Build history of the part. All positions in model axes, mm. Face numbers are marked on the shaded views. A direction names the side the tool comes from. Round coordinates to 2 decimals unless told otherwise and drop trailing zeros. Loops run counter-clockwise (first coordinate to the right, second up) from the corner with the lowest first, then second, coordinate; pieces in that order, holes last. Notation, with made-up numbers: (-11, 24) -> (41, 24) arc R35 cw to (41, 59) -> close; hole circle Ø8 at (-27, 84.25). An arc over 180 degrees is marked (long way). Put each result on its own line as item: value. Start each with the question number.
Item 1: Cut at B-B, the plane x = 156.5. List the corners of the cut face in (y, z), plus the area to 3 significant figures.
Item 2: Cut at A-A, the plane y = 334. List the corners of the cut face in (x, z), plus the area to 3 significant figures.
Item 3: Cut at C-C, the plane z = 1.45. List the corners of the cut face in (x, y).
Item 4: Tool access for the marked faces 1 and 2: list every direction of +Z, -Z, +X, -X, +Y, -Y with a clear straight run to the whole face (end or side of a thin tool).
Item 5: Cut at D-D, the plane y = 355. List the corners of the cut face in (x, z).
Item 6: Flat gauge pins, fed straight in: pin 1 Ø8 at (x, y) = (145.5, 366) entering from +Z; pin 2 Ø1.5 at (y, z) = (352.5, 0.5) entering from -X; pin 3 Ø1.5 at (x, z) = (157, 0.5) entering from +Y. Where does each tip first touch, or does it go through?
Item 7: Drill centre lines: probe 1 along X at (y, z) = (363, 0.35); probe 2 along Z at (x, y) = (118, 332.5); probe 3 along X at (y, z) = (361.5, 1.6). Where is each one in solid material? Low to high. Write a range as [from, to].
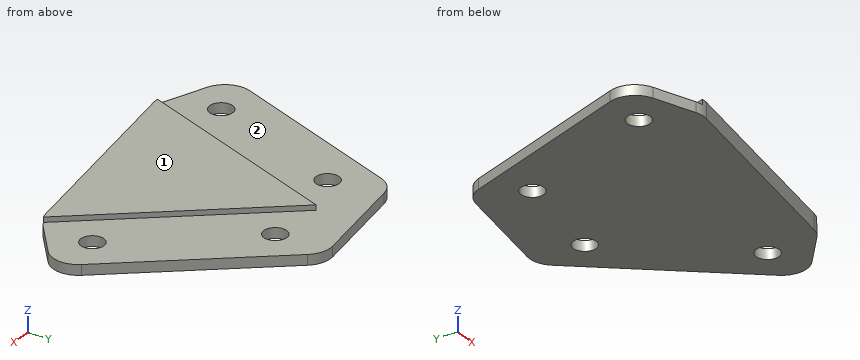
```python
from build123d import *

# Parameters (mm, degrees)
EXTRUDE_1_DEPTH     = 3
SKETCH_2_R          = 2.25
CUT_EXTRUDE_1_DEPTH = 3
FILLET_1_R          = 5
CUT_EXTRUDE_2_DEPTH = 1


with BuildPart() as part:
    # ｽｹｯﾁ1 → ﾎﾞｽ - 押し出し1 (new body)
    with BuildSketch(Plane.XY):
        Polygon((173.531323483, 340.900859956), (144.605881047, 375.372859896), (133.1152144, 365.731045751), (119.019825089, 370.861347901), (103.628918639, 328.575179965), (117.724307951, 323.444877815), (162.040656836, 331.259045811), align=None)
        Polygon((144.605881047, 375.372859896), (133.1152144, 365.731045751), (119.019825089, 370.861347901), align=None)
    extrude(amount=EXTRUDE_1_DEPTH)

    # ｽｹｯﾁ2 → ｶｯﾄ - 押し出し1 (cut)
    with BuildSketch(Plane.XY.offset(3)):
        with Locations((113.24176437, 333.057723546)):
            Circle(SKETCH_2_R)
        with Locations((123.50236867, 361.24850217)):
            Circle(SKETCH_2_R)
        with Locations((143.681454796, 364.8066195)):
            Circle(SKETCH_2_R)
        with Locations((162.965083087, 341.825286207)):
            Circle(SKETCH_2_R)
    extrude(amount=-CUT_EXTRUDE_1_DEPTH, mode=Mode.SUBTRACT)

    # ﾌｨﾚｯﾄ1
    fillet_1_edges = [part.edges().sort_by_distance(p)[0] for p in [
        (173.531323483, 340.900859956, 1.5),
        (162.040656836, 331.259045811, 1.5),
        (117.724307951, 323.444877815, 1.5),
        (103.628918639, 328.575179965, 1.5),
        (119.019825089, 370.861347901, 1.5),
        (144.605881047, 375.372859896, 1.5),
    ]]
    fillet(fillet_1_edges, radius=FILLET_1_R)

    # ｽｹｯﾁ3 → ｶｯﾄ - 押し出し2 (cut)
    with BuildSketch(Plane.XY.offset(3)):
        Polygon((121.413966092, 377.439196246), (103.628918639, 328.575179965), (117.771292582, 323.427776808), (133.132579218, 365.632564976), (162.002354614, 331.22690643), (173.531323483, 340.900859956), (140.106367779, 380.735170998), (131.711632891, 373.691152049), align=None)
    extrude(amount=-CUT_EXTRUDE_2_DEPTH, mode=Mode.SUBTRACT)


solid = part.part
```
Reply:
1. outline: (330.28, 0) -> (361.2, 0) -> (361.2, 2) -> (337.78, 2) -> (337.78, 3) -> (330.28, 3) -> close
1. area: 69.3 mm^2
2. outline: (105.6, 0) -> (111.2, 0) -> (111.2, 2) -> (105.6, 2) -> close; (115.28, 0) -> (165.31, 0) -> (165.31, 2) -> (159.68, 2) -> (159.68, 3) -> (121.62, 3) -> (121.62, 2) -> (115.28, 2) -> close
2. area: 149 mm^2
3. outline: (105.34, 333.27) arc R5 ccw to (108.33, 326.87) -> (116.47, 323.9) arc R5 ccw to (119.04, 323.68) -> (160.72, 331.03) arc R5 ccw to (163.07, 332.12) -> (169.7, 337.69) arc R5 ccw to (170.32, 344.73) -> (146.46, 373.16) arc R5 ccw to (141.76, 374.87) -> (121.86, 371.36) arc R5 ccw to (118.03, 368.15) -> close; hole circle Ø4.5 at (113.24, 333.06); hole circle Ø4.5 at (123.5, 361.25); hole circle Ø4.5 at (143.68, 364.81); hole circle Ø4.5 at (162.97, 341.83)
4. face 1: +Z, +X, -X, +Y, -Y
4. face 2: +Z, +Y
5. outline: (113.25, 0) -> (161.7, 0) -> (161.7, 2) -> (142.05, 2) -> (142.05, 3) -> (129.26, 3) -> (129.26, 2) -> (113.25, 2) -> close
6. pin 1: stops at z = 2
6. pin 2: stops at x = 112.06
6. pin 3: stops at y = 361.5
7. probe 1: x = [116.16, 122.09], [124.91, 142.34], [145.02, 154.99]
7. probe 2: z = [0, 2]
7. probe 3: x = [115.61, 121.27], [125.74, 156.25]
